The drawing under review shows one solid part. Ordinate dimensions are in mm from its lowest x, y, z. A direction names the side the tool comes from. Give positions to 0.01 mm unless a question says otherwise; leave off trailing zeros. Loops run counter-clockwise (first coordinate to the right, second up) from the corner with the lowest first, then second, coordinate; pieces in that order, holes last. Notation, with made-up numbers: M -2,-31.5 L 49,-31.5 A34 cw 49,5.5 Z; hole C 52.5,-37.75 d1. An arc over 180 degrees is marked long. Answer as CSV lines item,"result".
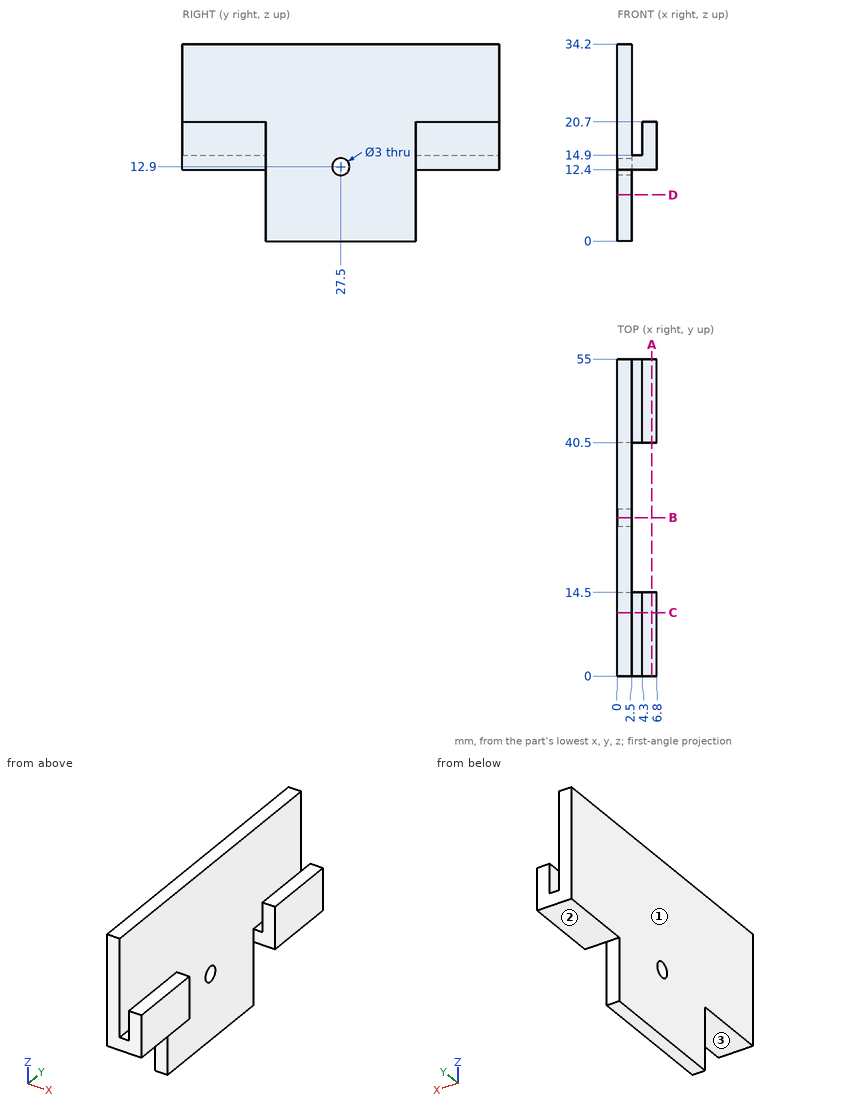
1. We need section D-D, the plane z = 8. Write out the cut boundary in (x, y).
Answer block:
outline,"M 0,14.5 L 2.5,14.5 L 2.5,40.5 L 0,40.5 Z"
2. To check wall thickness, follow L1, parallel to Y at x = 1.4, z = 12.9; L2, parallel to X at y = 41.5, z = 16.5; L3, parallel to X at y = 23, z = 7. State the ranges of each line that lie inside material, in increasing order. Write a range as [from, to].
Answer block:
L1,"[0, 26], [29, 55]"
L2,"[0, 2.5], [4.3, 6.8]"
L3,"[0, 2.5]"
3. We need section B-B, the plane y = 27.5. Write out the cut boundary in (x, z).
Answer block:
outline,"M 0,0 L 2.5,0 L 2.5,11.4 L 0,11.4 Z; M 0,14.4 L 2.5,14.4 L 2.5,34.2 L 0,34.2 Z"
4. For the marked faces 1, 2 and 3, list the 3-axis set-ups (+Z, -Z, +X, -X, +Y, -Y) from which the entire face can be reached by the end or side of a thin tool; tool diameter is ignored.
Answer block:
face 1,"+Z, -Z, -X, +Y, -Y"
face 2,"-Z, +X, -X, +Y"
face 3,"-Z, +X, -X, -Y"
5. We need section C-C, the plane y = 11. Write out the cut boundary in (x, z), plus the area to 4 significant figures.
Answer block:
outline,"M 0,12.4 L 6.8,12.4 L 6.8,20.7 L 4.3,20.7 L 4.3,14.9 L 2.5,14.9 L 2.5,34.2 L 0,34.2 Z"
area,"79.75 mm²"
6. For P1, Ø6, axis at y = 35.5, z = 12.5, coming from the -X side; P2, Ø1.2, axis at x = 1.5, z = 4.5, coming from the +Y side; P3, Ø6, axis at y = 34, z = 20.5, coming from the +X side; P4, Ø2, axis at x = 5, y = 11.5, coming from the -Z side, all flat-tipped, find the tip position at first contact; note any pin that passes through.
Answer block:
P1,"x = 0"
P2,"y = 40.5"
P3,"x = 2.5"
P4,"z = 12.4"
7. We need section A-A, the plane x = 6. Write out the cut boundary in (y, z), plus the area to 3 significant figures.
Answer block:
outline,"M 0,12.4 L 14.5,12.4 L 14.5,20.7 L 0,20.7 Z; M 40.5,12.4 L 55,12.4 L 55,20.7 L 40.5,20.7 Z"
area,"241 mm²"
